Here's how the part is built. I have some questions about the finished solid (model axes, mm). Face numbers are marked on the shaded views. Coordinates: 2 decimals unless noted, no trailing zeros. Write each loop counter-clockwise with the first axis right and the second up, starting at its lowest first coordinate (ties: lowest second). Pieces come first, ordered by that corner, then holes. Notation, with made-up numbers: M 34.25,-25.75 L 92.25,-25.75 A19 ccw 92.25,5.25 Z; hole C 69,-25.5 d3. An arc over 180 degrees is marked long. Use one line per item in the form item = value. Start each with the question number.
1. I want a section at A-A, the plane z = 0. List the corners of the cut face in (x, y) for me.
2. I want a section at B-B, the plane x = 0. List the corners of the cut face in (y, z) for me, plus the area to 3 significant figures.
3. I want a section at C-C, the plane x = -22. List the corners of the cut face in (y, z) for me, plus the area to 3 significant figures.
4. I want a section at D-D, the plane z = 33.5. List the corners of the cut face in (x, y) for me, plus the area to 3 significant figures.
5. Please list where these lines run through material, in increasing order: line 1 along X through (y, z) = (3.5, 0); line 2 along X through (y, z) = (6.1, 0); line 3 along Y through (x, z) = (37, -18.5). Write a range as [from, to].
6. I'm going to push flat-ended pins straight in: pin 1 Ø5 at (x, z) = (-33.5, 20.5) entering from +Y; pin 2 Ø4.5 at (x, z) = (-21.5, 1) entering from +Y; pin 3 Ø3 at (y, z) = (3.5, -28) entering from -X; pin 4 Ø2.5 at (x, z) = (-22, 0) entering from -Y. Where does each tip first touch, or does it pass through?
7. Thinking about a two-plate mould opening in X: for the marked faces 1, 2 and 3, which applies, released by +X, released by -X, zero draft, split by the parting line, or undercut?
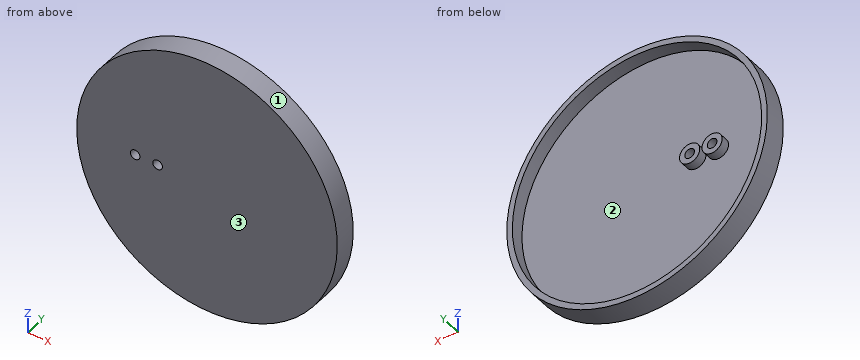
from build123d import *

# Parameters (mm, degrees)
SKETCH_1_R                       = 4.5
MOVING_POST_A_DEPTH              = 8
SKETCH_2_R                       = 58
CUP_PLATE_D116_T4_DEPTH          = 4
SKETCH_3_R                       = 4.5
MOVING_POST_B_DEPTH              = 8
SKETCH_4_R                       = 58
SKETCH_4_R_2                     = 55.5
DRIP_SKIRT_OD116_ID111_H10_DEPTH = 10
SKETCH_5_R                       = 2.15
M4_MOVING_MOUNT_CLEARANCE_DEPTH  = 8


with BuildPart() as part:
    # 草图1 → Moving_post_A (new body)
    with BuildSketch(Plane(origin=(0, 0, 0), x_dir=(1, 0, 0), z_dir=(0, 1, 0))):
        with Locations(Location((-22, 0, 0), (0, 0, 270))):
            Circle(SKETCH_1_R)
    extrude(amount=MOVING_POST_A_DEPTH)

    # 草图2 → Cup_plate_D116_T4 (add)
    with BuildSketch(Plane(origin=(0, 0, 0), x_dir=(1, 0, 0), z_dir=(0, 1, 0))):
        with Locations(Location((0, 0, 0), (0, 0, 270))):
            Circle(SKETCH_2_R)
    extrude(amount=CUP_PLATE_D116_T4_DEPTH)

    # 草图3 → Moving_post_B (add)
    with BuildSketch(Plane(origin=(0, 0, 0), x_dir=(1, 0, 0), z_dir=(0, 1, 0))):
        with Locations(Location((-32, 0, 0), (0, 0, 270))):
            Circle(SKETCH_3_R)
    extrude(amount=MOVING_POST_B_DEPTH)

    # 草图4 → Drip_skirt_OD116_ID111_H10 (add)
    with BuildSketch(Plane(origin=(0, 0, 0), x_dir=(1, 0, 0), z_dir=(0, 1, 0))):
        with Locations(Location((0, 0, 0), (0, 0, 270))):
            Circle(SKETCH_4_R)
        with Locations(Location((0, 0, 0), (0, 0, 270))):
            Circle(SKETCH_4_R_2, mode=Mode.SUBTRACT)
    extrude(amount=DRIP_SKIRT_OD116_ID111_H10_DEPTH)

    # 草图5 → M4_moving_mount_clearance (cut)
    with BuildSketch(Plane(origin=(0, 0, 0), x_dir=(1, 0, 0), z_dir=(0, 1, 0))):
        with Locations(Location((-22, 0, 0), (0, 0, 270))):
            Circle(SKETCH_5_R)
        with Locations(Location((-32, 0, 0), (0, 0, 270))):
            Circle(SKETCH_5_R)
    extrude(amount=M4_MOVING_MOUNT_CLEARANCE_DEPTH, mode=Mode.SUBTRACT)


solid = part.part
Answer list:
q1.outline = M -58,0 L -34.15,0 L -34.15,8 L -36.5,8 L -36.5,4 L -55.5,4 L -55.5,10 L -58,10 Z; M -29.85,0 L -24.15,0 L -24.15,8 L -26.5,8 L -26.5,4 L -27.5,4 L -27.5,8 L -29.85,8 Z; M -19.85,0 L 58,0 L 58,10 L 55.5,10 L 55.5,4 L -17.5,4 L -17.5,8 L -19.85,8 Z
q2.outline = M 0,-58 L 10,-58 L 10,-55.5 L 4,-55.5 L 4,55.5 L 10,55.5 L 10,58 L 0,58 Z
q2.area = 494 mm²
q3.outline = M 0,-53.67 L 10,-53.67 L 10,-50.95 L 4,-50.95 L 4,-4.5 L 8,-4.5 L 8,-2.15 L 0,-2.15 Z; M 0,2.15 L 8,2.15 L 8,4.5 L 4,4.5 L 4,50.95 L 10,50.95 L 10,53.67 L 0,53.67 Z
q3.area = 463 mm²
q4.outline = M -47.35,0 L 47.35,0 L 47.35,10 L 44.25,10 L 44.25,4 L -44.25,4 L -44.25,10 L -47.35,10 Z
q4.area = 416 mm²
q5.line_1 = [-58, -34.15], [-29.85, -24.15], [-19.85, 58]
q5.line_2 = [-58, -55.5], [-36.5, -34.15], [-29.85, -27.5], [-26.5, -24.15], [-19.85, -17.5], [55.5, 58]
q5.line_3 = [0, 4]
q6.pin_1 = 4
q6.pin_2 = 8
q6.pin_3 = -51.59
q6.pin_4 = through
q7.face_1 = split by the parting line
q7.face_2 = undercut
q7.face_3 = zero draft
